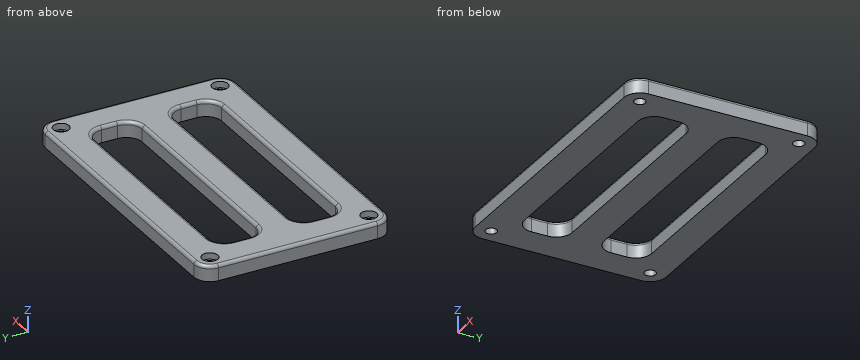
from build123d import *

# Parameters (mm, degrees)
SKETCH1_W           = 95
SKETCH1_H           = 60
SKETCH1_W_2         = 75
SKETCH1_H_2         = 40
BOSS_EXTRUDE1_DEPTH = 5
BOSS_EXTRUDE2_DEPTH = 5
SKETCH5_R           = 1.75
CUT_EXTRUDE2_DEPTH  = 99.742088291
SKETCH6_R           = 2.5
CUT_EXTRUDE3_DEPTH  = 2
FILLET1_R           = 5
FILLET2_R           = 1


with BuildPart() as part:
    # Sketch1 → Boss-Extrude1 (new body)
    with BuildSketch(Plane.XY):
        with Locations((37.5, 20)):
            Rectangle(SKETCH1_W, SKETCH1_H)
        with Locations((37.5, 20)):
            Rectangle(SKETCH1_W_2, SKETCH1_H_2, mode=Mode.SUBTRACT)
    extrude(amount=BOSS_EXTRUDE1_DEPTH)

    # Sketch2 → Boss-Extrude2 (add)
    with BuildSketch(Plane.XY.offset(5)):
        Polygon((0, 25), (75, 25), (75, 20), (75, 15), (0, 15), (0, 20), align=None)
    extrude(amount=-BOSS_EXTRUDE2_DEPTH)

    # Sketch5 → Cut-Extrude2 (cut, through all)
    with BuildSketch(Plane.XY.offset(5)):
        with Locations((-5, 45)):
            Circle(SKETCH5_R)
        with Locations((80, 45)):
            Circle(SKETCH5_R)
        with Locations((80, -5)):
            Circle(SKETCH5_R)
        with Locations((-5, -5)):
            Circle(SKETCH5_R)
    extrude(amount=-CUT_EXTRUDE2_DEPTH, mode=Mode.SUBTRACT)

    # Sketch6 → Cut-Extrude3 (cut)
    with BuildSketch(Plane.XY.offset(5)):
        with Locations((-5, 45)):
            Circle(SKETCH6_R)
        with Locations((80, 45)):
            Circle(SKETCH6_R)
        with Locations((80, -5)):
            Circle(SKETCH6_R)
        with Locations((-5, -5)):
            Circle(SKETCH6_R)
    extrude(amount=-CUT_EXTRUDE3_DEPTH, mode=Mode.SUBTRACT)

    # Fillet1
    fillet1_edges = [part.edges().sort_by_distance(p)[0] for p in [
        (0, 40, 2.5),
        (0, 0, 2.5),
        (75, 0, 2.5),
        (75, 40, 2.5),
        (0, 15, 2.5),
        (0, 25, 2.5),
        (75, 25, 2.5),
        (75, 15, 2.5),
        (-10, 50, 2.5),
        (85, 50, 2.5),
        (85, -10, 2.5),
        (-10, -10, 2.5),
    ]]
    fillet(fillet1_edges, radius=FILLET1_R)

    # Fillet2
    fillet2_edges = [part.edges().sort_by_distance(p)[0] for p in [
        (0, 7.5, 5),
        (37.5, 15, 5),
        (37.5, 0, 5),
        (75, 7.5, 5),
        (37.5, 25, 5),
        (0, 32.5, 5),
        (75, 32.5, 5),
        (37.5, 40, 5),
        (-10, 20, 5),
        (37.5, 50, 5),
        (37.5, -10, 5),
        (85, 20, 5),
        (-8.535533906, -8.535533906, 5),
        (83.535533906, -8.535533906, 5),
        (83.535533906, 48.535533906, 5),
        (-8.535533906, 48.535533906, 5),
        (1.464466094, 13.535533906, 5),
        (73.535533906, 1.464466094, 5),
        (73.535533906, 13.535533906, 5),
        (1.464466094, 1.464466094, 5),
        (1.464466094, 26.464466094, 5),
        (73.535533906, 26.464466094, 5),
        (73.535533906, 38.535533906, 5),
        (1.464466094, 38.535533906, 5),
    ]]
    fillet(fillet2_edges, radius=FILLET2_R)


solid = part.part
Design review of the part built by this model. Coordinates are the model's own, in mm. Coordinates: 2 decimals unless noted, no trailing zeros. Loops run counter-clockwise (first coordinate to the right, second up) from the corner with the lowest first, then second, coordinate; pieces in that order, holes last.
Item 1: Add section B-B (x = 21). Write out the cut boundary in (y, z), and give its area (3 significant figures).
Completed:
outline: (-10, 0) - (0, 0) - (0, 4) arc R1 ccw to (-1, 5) - (-9, 5) arc R1 ccw to (-10, 4) - close; (15, 0) - (25, 0) - (25, 4) arc R1 ccw to (24, 5) - (16, 5) arc R1 ccw to (15, 4) - close; (40, 0) - (50, 0) - (50, 4) arc R1 ccw to (49, 5) - (41, 5) arc R1 ccw to (40, 4) - close
area: 149 mm2
Item 2: Add section A-A (z = 1.3). Write out the cut boundary in (x, y).
Completed:
outline: (-10, -5) arc R5 ccw to (-5, -10) - (80, -10) arc R5 ccw to (85, -5) - (85, 45) arc R5 ccw to (80, 50) - (-5, 50) arc R5 ccw to (-10, 45) - close; hole circle Ø3.5 at (-5, -5); hole circle Ø3.5 at (-5, 45); hole (0, 5) arc R5 ccw to (5, 0) - (70, 0) arc R5 ccw to (75, 5) - (75, 10) arc R5 ccw to (70, 15) - (5, 15) arc R5 ccw to (0, 10) - close; hole (0, 30) arc R5 ccw to (5, 25) - (70, 25) arc R5 ccw to (75, 30) - (75, 35) arc R5 ccw to (70, 40) - (5, 40) arc R5 ccw to (0, 35) - close; hole circle Ø3.5 at (80, -5); hole circle Ø3.5 at (80, 45)
Item 3: Wall thickness on L1, parallel to Y at x = 80, z = 1.15; L2, parallel to Y at x = -5, z = 3.9; L3, parallel to X at y = 9.5, z = 0.8: over which ranges is each line inside the solid? List them lowest first.
Completed:
L1: y = -10 to -6.75, -3.25 to 43.25, 46.75 to 50
L2: y = -10 to -7.5, -2.5 to 42.5, 47.5 to 50
L3: x = -10 to 0, 75 to 85
Item 4: Clearance check with flat-ended pins moving along their axes: pin 1 (8 mm diameter, centred on x = 70.5, y = 32.5, fed in from -Z); pin 2 (4 mm diameter, centred on x = 80, y = -5, fed in from +Z). State where each tip first meets the part, or that it passes through.
Completed:
pin 1: passes through
pin 2: stops at z = 3
